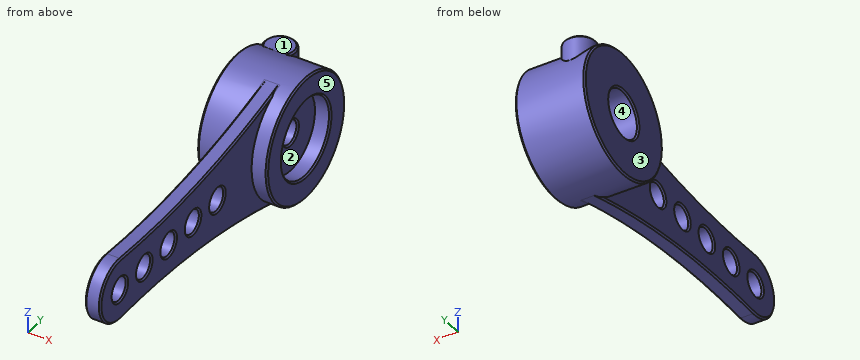
from build123d import *

# Parameters (mm, degrees)
SKETCH_1_R          = 8
EXTRUDE_1_DEPTH     = 9
SKETCH_2_R          = 5
CUT_EXTRUDE_1_DEPTH = 2
SKETCH_3_R          = 1.5
CUT_EXTRUDE_2_DEPTH = 2
SKETCH_4_R          = 3
CUT_EXTRUDE_3_DEPTH = 5
SKETCH_6_R          = 2
EXTRUDE_2_DEPTH     = 7
SKETCH_7_R          = 1.5
EXTRUDE_3_DEPTH     = 2
CHAMFER_1_SIZE      = 0.2
CHAMFER_2_SIZE      = 0.2


with BuildPart() as part:
    # 草图1 → 凸台-拉伸1 (new body)
    with BuildSketch(Plane(origin=(0, 0, 0), x_dir=(0, 0, -1), z_dir=(1, 0, 0))):
        Circle(SKETCH_1_R)
    extrude(amount=EXTRUDE_1_DEPTH)

    # 草图2 → 切除-拉伸1 (cut)
    with BuildSketch(Plane(origin=(9, 0, 0), x_dir=(0, 0, -1), z_dir=(1, 0, 0))):
        Circle(SKETCH_2_R)
    extrude(amount=-CUT_EXTRUDE_1_DEPTH, mode=Mode.SUBTRACT)

    # 草图3 → 切除-拉伸2 (cut)
    with BuildSketch(Plane(origin=(7, 0, 0), x_dir=(0, 0, -1), z_dir=(1, 0, 0))):
        Circle(SKETCH_3_R)
    extrude(amount=-CUT_EXTRUDE_2_DEPTH, mode=Mode.SUBTRACT)

    # 草图4 → 切除-拉伸3 (cut)
    with BuildSketch(Plane(origin=(5, 0, 0), x_dir=(0, 0, -1), z_dir=(1, 0, 0))):
        Circle(SKETCH_4_R)
    extrude(amount=-CUT_EXTRUDE_3_DEPTH, mode=Mode.SUBTRACT)

    # 草图6 → 凸台-拉伸2 (add)
    with BuildSketch(Plane.XY):
        with Locations((2.5, 5)):
            Circle(SKETCH_6_R)
    extrude(amount=EXTRUDE_2_DEPTH)

    # 草图7 → 凸台-拉伸3 (add)
    with BuildSketch(Plane.ZY.offset(-5)):
        with BuildLine():
            ThreePointArc((-3.994632879, -34.792857143), (0, -39), (3.994632879, -34.792857143))
            ThreePointArc((3.994632879, -34.792857143), (4.497974535, -18.34053276), (7.693367026, -2.193650794))
            ThreePointArc((7.693367026, -2.193650794), (0, -8), (-7.693367026, -2.193650794))
            ThreePointArc((-7.693367026, -2.193650794), (-4.497974535, -18.34053276), (-3.994632879, -34.792857143))
        make_face()
        with Locations((0, -35)):
            Circle(SKETCH_7_R, mode=Mode.SUBTRACT)
        with Locations((0, -30)):
            Circle(SKETCH_7_R, mode=Mode.SUBTRACT)
        with Locations((0, -25)):
            Circle(SKETCH_7_R, mode=Mode.SUBTRACT)
        with Locations((0, -20)):
            Circle(SKETCH_7_R, mode=Mode.SUBTRACT)
        with Locations((0, -15)):
            Circle(SKETCH_7_R, mode=Mode.SUBTRACT)
    extrude(amount=-EXTRUDE_3_DEPTH)

    # 倒角1
    # the kernel refuses this chamfer: 0.2 mm, written as the material it takes off along each edge
    with BuildSketch(Plane(origin=(2.5, 5, 7), x_dir=(0.6550221051171238, -0.7556097152683597, 0), z_dir=(-0.7556097152683597, -0.6550221051171238, 0))) as chamfer_1_piece_1_section:
        Polygon((2 - CHAMFER_1_SIZE, 0), (2, -CHAMFER_1_SIZE), (2, 0), align=None)
    chamfer_1_piece_1 = revolve(axis=Axis((2.5, 5, 7), (0, 0, 1)), revolution_arc=278.157347794, mode=Mode.PRIVATE)
    chamfer_1_piece_1 = chamfer_1_piece_1 - Plane(origin=(2.5, 0, 0), x_dir=(0, 0, -1), z_dir=(-1, 0, 0)) * Cylinder(8, 9, mode=Mode.PRIVATE)
    add(chamfer_1_piece_1, mode=Mode.SUBTRACT)
    with BuildSketch(Plane(origin=(0, 0, 0), x_dir=(0, 0, -1), z_dir=(0, -1, 0))) as chamfer_1_piece_2:
        Polygon((3 + CHAMFER_1_SIZE, 0), (3, CHAMFER_1_SIZE), (3, 0), align=None)
    revolve(axis=Axis((0, 0, 0), (1, 0, 0)), mode=Mode.SUBTRACT)
    with BuildSketch(Plane(origin=(0, 0, 0), x_dir=(0, 0, -1), z_dir=(0, -1, 0))) as chamfer_1_piece_3:
        Polygon((8, CHAMFER_1_SIZE), (8 - CHAMFER_1_SIZE, 0), (8, 0), align=None)
    revolve(axis=Axis((0, 0, 0), (1, 0, 0)), mode=Mode.SUBTRACT)
    with BuildSketch(Plane(origin=(7, 0, 0), x_dir=(0, 0, -1), z_dir=(0, -1, 0))) as chamfer_1_piece_4:
        Polygon((1.5 + CHAMFER_1_SIZE, 0), (1.5, -CHAMFER_1_SIZE), (1.5, 0), align=None)
    revolve(axis=Axis((7, 0, 0), (1, 0, 0)), mode=Mode.SUBTRACT)
    with BuildSketch(Plane(origin=(9, 0, 0), x_dir=(0, 0, -1), z_dir=(0, -1, 0))) as chamfer_1_piece_5:
        Polygon((5 + CHAMFER_1_SIZE, 0), (5, -CHAMFER_1_SIZE), (5, 0), align=None)
    revolve(axis=Axis((9, 0, 0), (1, 0, 0)), mode=Mode.SUBTRACT)
    with BuildSketch(Plane(origin=(9, 0, 0), x_dir=(0, 0, -1), z_dir=(0, -1, 0))) as chamfer_1_piece_6:
        Polygon((8, -CHAMFER_1_SIZE), (8 - CHAMFER_1_SIZE, 0), (8, 0), align=None)
    revolve(axis=Axis((9, 0, 0), (1, 0, 0)), mode=Mode.SUBTRACT)

    # 倒角2
    # the kernel refuses this chamfer: 0.2 mm, written as the material it takes off along each edge
    with BuildSketch(Plane(origin=(7, -29.614285714, 103.86045485), x_dir=(0, -0.05178571428571552, -0.9986582197107868), z_dir=(0, -0.9986582197107868, 0.05178571428571552))) as chamfer_2_piece_1_section:
        Polygon((100, -CHAMFER_2_SIZE), (100 + CHAMFER_2_SIZE, 0), (100, 0), align=None)
    chamfer_2_piece_1 = revolve(axis=Axis((7, -29.614285714, 103.86045485), (1, 0, 0)), revolution_arc=20.356645861, mode=Mode.PRIVATE)
    chamfer_2_piece_1 = chamfer_2_piece_1 - Plane(origin=(7, 0, 0), x_dir=(0, 0, -1), z_dir=(-1, 0, 0)) * Cylinder(8, 401, mode=Mode.PRIVATE)
    add(chamfer_2_piece_1, mode=Mode.SUBTRACT)
    with BuildSketch(Plane(origin=(7, -35, 0), x_dir=(0, 0.05178571428571369, -0.9986582197107869), z_dir=(0, 0.9986582197107869, 0.05178571428571369))) as chamfer_2_piece_2:
        Polygon((4 - CHAMFER_2_SIZE, 0), (4, CHAMFER_2_SIZE), (4, 0), align=None)
    revolve(axis=Axis((7, -35, 0), (-1, 0, 0)), revolution_arc=185.936861294, mode=Mode.SUBTRACT)
    with BuildSketch(Plane(origin=(7, -29.614285714, -103.86045485), x_dir=(0, 0.29884451461423694, 0.9543018160335759), z_dir=(0, 0.9543018160335759, -0.29884451461423694))) as chamfer_2_piece_3_section:
        Polygon((100 + CHAMFER_2_SIZE, 0), (100, -CHAMFER_2_SIZE), (100, 0), align=None)
    chamfer_2_piece_3 = revolve(axis=Axis((7, -29.614285714, -103.86045485), (1, 0, 0)), revolution_arc=20.356645861, mode=Mode.PRIVATE)
    chamfer_2_piece_3 = chamfer_2_piece_3 - Plane(origin=(7, 0, 0), x_dir=(0, 0, -1), z_dir=(-1, 0, 0)) * Cylinder(8, 401, mode=Mode.PRIVATE)
    add(chamfer_2_piece_3, mode=Mode.SUBTRACT)
    with BuildSketch(Plane(origin=(7, -15, 0), x_dir=(0, 0, 1), z_dir=(0, -1, 0))) as chamfer_2_piece_4:
        Polygon((1.5 + CHAMFER_2_SIZE, 0), (1.5, CHAMFER_2_SIZE), (1.5, 0), align=None)
    revolve(axis=Axis((7, -15, 0), (-1, 0, 0)), mode=Mode.SUBTRACT)
    with BuildSketch(Plane(origin=(7, -20, 0), x_dir=(0, 0, 1), z_dir=(0, -1, 0))) as chamfer_2_piece_5:
        Polygon((1.5 + CHAMFER_2_SIZE, 0), (1.5, CHAMFER_2_SIZE), (1.5, 0), align=None)
    revolve(axis=Axis((7, -20, 0), (-1, 0, 0)), mode=Mode.SUBTRACT)
    with BuildSketch(Plane(origin=(7, -25, 0), x_dir=(0, 0, 1), z_dir=(0, -1, 0))) as chamfer_2_piece_6:
        Polygon((1.5 + CHAMFER_2_SIZE, 0), (1.5, CHAMFER_2_SIZE), (1.5, 0), align=None)
    revolve(axis=Axis((7, -25, 0), (-1, 0, 0)), mode=Mode.SUBTRACT)
    with BuildSketch(Plane(origin=(7, -30, 0), x_dir=(0, 0, 1), z_dir=(0, -1, 0))) as chamfer_2_piece_7:
        Polygon((1.5 + CHAMFER_2_SIZE, 0), (1.5, CHAMFER_2_SIZE), (1.5, 0), align=None)
    revolve(axis=Axis((7, -30, 0), (-1, 0, 0)), mode=Mode.SUBTRACT)
    with BuildSketch(Plane(origin=(7, -35, 0), x_dir=(0, 0, 1), z_dir=(0, -1, 0))) as chamfer_2_piece_8:
        Polygon((1.5 + CHAMFER_2_SIZE, 0), (1.5, CHAMFER_2_SIZE), (1.5, 0), align=None)
    revolve(axis=Axis((7, -35, 0), (-1, 0, 0)), mode=Mode.SUBTRACT)
    with BuildSketch(Plane(origin=(5, -29.614285714, -103.86045485), x_dir=(0, 0.29884451461423694, 0.9543018160335759), z_dir=(0, 0.9543018160335759, -0.29884451461423694))) as chamfer_2_piece_9_section:
        Polygon((100 + CHAMFER_2_SIZE, 0), (100, CHAMFER_2_SIZE), (100, 0), align=None)
    chamfer_2_piece_9 = revolve(axis=Axis((5, -29.614285714, -103.86045485), (1, 0, 0)), revolution_arc=20.356645861, mode=Mode.PRIVATE)
    chamfer_2_piece_9 = chamfer_2_piece_9 - Plane(origin=(5, 0, 0), x_dir=(0, 0, -1), z_dir=(-1, 0, 0)) * Cylinder(8, 401, mode=Mode.PRIVATE)
    add(chamfer_2_piece_9, mode=Mode.SUBTRACT)
    with BuildSketch(Plane(origin=(5, -35, 0), x_dir=(0, 0.05178571428571369, -0.9986582197107869), z_dir=(0, 0.9986582197107869, 0.05178571428571369))) as chamfer_2_piece_10:
        Polygon((4 - CHAMFER_2_SIZE, 0), (4, -CHAMFER_2_SIZE), (4, 0), align=None)
    revolve(axis=Axis((5, -35, 0), (-1, 0, 0)), revolution_arc=185.936861294, mode=Mode.SUBTRACT)
    with BuildSketch(Plane(origin=(5, -29.614285714, 103.86045485), x_dir=(0, -0.05178571428571552, -0.9986582197107868), z_dir=(0, -0.9986582197107868, 0.05178571428571552))) as chamfer_2_piece_11_section:
        Polygon((100, CHAMFER_2_SIZE), (100 + CHAMFER_2_SIZE, 0), (100, 0), align=None)
    chamfer_2_piece_11 = revolve(axis=Axis((5, -29.614285714, 103.86045485), (1, 0, 0)), revolution_arc=20.356645861, mode=Mode.PRIVATE)
    chamfer_2_piece_11 = chamfer_2_piece_11 - Plane(origin=(5, 0, 0), x_dir=(0, 0, -1), z_dir=(-1, 0, 0)) * Cylinder(8, 401, mode=Mode.PRIVATE)
    add(chamfer_2_piece_11, mode=Mode.SUBTRACT)
    with BuildSketch(Plane(origin=(5, -35, 0), x_dir=(0, 0, 1), z_dir=(0, -1, 0))) as chamfer_2_piece_12:
        Polygon((1.5 + CHAMFER_2_SIZE, 0), (1.5, -CHAMFER_2_SIZE), (1.5, 0), align=None)
    revolve(axis=Axis((5, -35, 0), (-1, 0, 0)), mode=Mode.SUBTRACT)
    with BuildSketch(Plane(origin=(5, -30, 0), x_dir=(0, 0, 1), z_dir=(0, -1, 0))) as chamfer_2_piece_13:
        Polygon((1.5 + CHAMFER_2_SIZE, 0), (1.5, -CHAMFER_2_SIZE), (1.5, 0), align=None)
    revolve(axis=Axis((5, -30, 0), (-1, 0, 0)), mode=Mode.SUBTRACT)
    with BuildSketch(Plane(origin=(5, -25, 0), x_dir=(0, 0, 1), z_dir=(0, -1, 0))) as chamfer_2_piece_14:
        Polygon((1.5 + CHAMFER_2_SIZE, 0), (1.5, -CHAMFER_2_SIZE), (1.5, 0), align=None)
    revolve(axis=Axis((5, -25, 0), (-1, 0, 0)), mode=Mode.SUBTRACT)
    with BuildSketch(Plane(origin=(5, -20, 0), x_dir=(0, 0, 1), z_dir=(0, -1, 0))) as chamfer_2_piece_15:
        Polygon((1.5 + CHAMFER_2_SIZE, 0), (1.5, -CHAMFER_2_SIZE), (1.5, 0), align=None)
    revolve(axis=Axis((5, -20, 0), (-1, 0, 0)), mode=Mode.SUBTRACT)
    with BuildSketch(Plane(origin=(5, -15, 0), x_dir=(0, 0, 1), z_dir=(0, -1, 0))) as chamfer_2_piece_16:
        Polygon((1.5 + CHAMFER_2_SIZE, 0), (1.5, -CHAMFER_2_SIZE), (1.5, 0), align=None)
    revolve(axis=Axis((5, -15, 0), (-1, 0, 0)), mode=Mode.SUBTRACT)


solid = part.part
For this review, take the finished solid that the model builds, in its own axes (mm). Face numbers are marked on the shaded views. A direction names the side the tool comes from. Give positions to 0.01 mm unless a question says otherwise; leave off trailing zeros. Order: outer loops, then holes, each group sorted by start corner. A loop starts at its lowest first (then second) coordinate and runs counter-clockwise, first axis right, second up. Notation, with made-up numbers: M -15,58 L 43,58 A15 cw 43,72 Z; hole C 54.5,-37.5 d10. An arc over 180 degrees is marked long. Answer in a Markdown table with one row per item. Add a question column.
(1) For pin 1 (3 mm diameter, centred on y = -11.5, z = 0.5, fed in from -X); pin 2 (3 mm diameter, centred on y = -29.5, z = -6, fed in from +X); pin 3 (0.9 mm diameter, centred on x = 3, y = 5, fed in from +Z); pin 4 (1 mm diameter, centred on x = 4, z = 2, fed in from -Y), all flat-tipped, find the tip position at first contact; note any pin that passes through.
(2) Wall thickness on probe 1 along Y at (x, z) = (2.3, 0); probe 2 along Y at (x, z) = (7.25, -4); probe 3 along Z at (x, y) = (4.5, 1): over which ranges is each line inside the solid? List them lowest first. Write a range as [from, to].
(3) Consider section A-A on y = 0. State the section outline as (x, z) points.
(4) For the marked faces 1, 2 and 3, list the 3-axis set-ups (+Z, -Z, +X, -X, +Y, -Y) from which the entire face can be reached by the end or side of a thin tool; tool diameter is ignored.
(5) Mouldability with a two-part tool opening along Y and no side actions: class the marked faces 4 and 5 as +Y half, -Y half, draft (parallel to the pull), parting line (faces both ways), or undercut.
(6) Consider section B-B on z = 0. Give the number of separate pieces and of enclosed holes in the cut face, and give its area (3 significant figures).
Evaluation:
| question | item | result |
|---|---|---|
| 1 | pin 1 | stops at x = 5 |
| 1 | pin 2 | passes through |
| 1 | pin 3 | stops at z = 7 |
| 1 | pin 4 | stops at y = -7.86 |
| 2 | probe 1 | y = [-8, -3], [3, 8] |
| 2 | probe 2 | y = [-6.93, -3], [3, 6.93] |
| 2 | probe 3 | z = [-7.94, -2.83], [2.83, 7.94] |
| 3 | outline | M 0,-7.8 L 0.2,-8 L 8.8,-8 L 9,-7.8 L 9,-5.2 L 8.8,-5 L 7,-5 L 7,-1.7 L 6.8,-1.5 L 5,-1.5 L 5,-3 L 0.2,-3 L 0,-3.2 Z; M 0,3.2 L 0.2,3 L 5,3 L 5,1.5 L 6.8,1.5 L 7,1.7 L 7,5 L 8.8,5 L 9,5.2 L 9,7.8 L 8.8,8 L 0.2,8 L 0,7.8 Z |
| 4 | face 1 | +Z, +X, -X, +Y |
| 4 | face 2 | +X |
| 4 | face 3 | +Z, -Z, -X, +Y, -Y |
| 5 | face 4 | undercut |
| 5 | face 5 | draft |
| 6 | separate pieces | 7 |
| 6 | enclosed holes | 0 |
| 6 | area | 119 mm^2 |
